Read the model definition and answer for the solid it produces. Units are mm, in the model's axes. Face numbers are marked on the shaded views. A direction names the side the tool comes from. Give positions to 0.01 mm unless a question says otherwise; leave off trailing zeros. Write each loop counter-clockwise with the first axis right and the second up, starting at its lowest first coordinate (ties: lowest second). Pieces come first, ordered by that corner, then holes. Notation, with made-up numbers: (3, -34) -> (45, -34) arc R16 ccw to (45, -7) -> close; hole circle Ø5 at (31, 82.5). An arc over 180 degrees is marked (long way). Use a Markdown table: item, result.
Autodesk Fusion 360 part; units mm, degrees
sketch "Sketch1" plane through (0, 0, 0) normal (0, 0, 1) x (1, 0, 0)
  line L0 (0, 0) -> (55, 0)
  line L1 (55, 0) -> (55, 50)
  line L2 (55, 50) -> (0, 50)
  line L3 (0, 50) -> (0, 0)
  dimension "d1" = 55
  dimension "d2" = 50
extrude "Extrude1" add sketch "Sketch1" along normal blind 5
sketch "Sketch2" plane through (0, 0, 5) normal (0, 0, 1) x (-1, 0, 0)
  line L0 (0, -50) -> (0, 0)
  line L1 (0, 0) -> (-55, 0)
  line L2 (-55, 0) -> (-55, -50)
  line L3 (-55, -50) -> (0, -50)
  circle A0 centre (-10, -40) radius 3
  circle A1 centre (-10, -10) radius 3
  circle A2 centre (-40, -10) radius 3
  circle A3 centre (-40, -40) radius 3
  dimension "d5" = 6
  dimension "d6" = 6
  dimension "d7" = 6
  dimension "d8" = 6
extrude "Extrude2" cut sketch "Sketch2" against normal blind 5 contours A0 | A1 | A2 | A3
sketch "Sketch3" plane through (0, 0, 5) normal (0, 0, 1) x (-1, 0, 0)
  circle A0 centre (-40, -40) radius 3
  circle A1 centre (-40, -10) radius 3
  circle A2 centre (-10, -40) radius 3
  circle A3 centre (-10, -10) radius 3
  line L0 (0, -50) -> (0, 0)
  line L1 (0, 0) -> (-55, 0)
  line L2 (-55, 0) -> (-55, -50)
  line L3 (-55, -50) -> (0, -50)
  circle A4 centre (-10, -10) radius 5
  circle A5 centre (-10, -40) radius 5
  circle A6 centre (-40, -40) radius 5
  circle A7 centre (-40, -10) radius 5
  dimension "d11" = 10
  dimension "d12" = 10
  dimension "d13" = 10
  dimension "d14" = 10
extrude "Extrude3" cut sketch "Sketch3" against normal blind 2 contours A4 | A5 | A6 | A7
sketch "Sketch4" plane through (0, 0, 5) normal (0, 0, 1) x (-1, 0, 0)
  circle A0 centre (-40, -40) radius 5
  circle A1 centre (-40, -10) radius 5
  circle A2 centre (-10, -40) radius 5
  circle A3 centre (-10, -10) radius 5
  line L0 (0, -50) -> (0, 0)
  line L1 (0, 0) -> (-55, 0)
  line L2 (-55, 0) -> (-55, -50)
  line L3 (-55, -50) -> (0, -50)
  line L4 (-50, 0) -> (-55, 0)
  line L5 (-55, 0) -> (-55, -50)
  line L6 (-55, -50) -> (-50, -50)
  line L7 (-50, -50) -> (-50, 0)
  dimension "d17" = 5
  dimension "d18" = 50
extrude "Extrude4" add sketch "Sketch4" along normal blind 50 contours L1 L2 L3 L4 L5 L6 L7
sketch "Sketch5" plane through (50, 0, 0) normal (-1, 0, 0) x (0, -1, 0)
  line L0 (-50, 5) -> (0, 5)
  line L1 (0, 5) -> (0, 55)
  line L2 (0, 55) -> (-50, 55)
  line L3 (-50, 55) -> (-50, 5)
  circle A0 centre (-40, 45) radius 3
  circle A1 centre (-10, 45) radius 3
  circle A2 centre (-10, 15) radius 3
  circle A3 centre (-40, 15) radius 3
  dimension "d21" = 6
  dimension "d22" = 6
  dimension "d23" = 6
  dimension "d24" = 6
extrude "Extrude5" cut sketch "Sketch5" against normal blind 5 contours A0 | A1 | A2 | A3
sketch "Sketch6" plane through (50, 0, 0) normal (-1, 0, 0) x (0, -1, 0)
  circle A0 centre (-10, 45) radius 3
  circle A1 centre (-10, 15) radius 3
  circle A2 centre (-40, 45) radius 3
  circle A3 centre (-40, 15) radius 3
  line L0 (-50, 5) -> (0, 5)
  line L1 (0, 5) -> (0, 55)
  line L2 (0, 55) -> (-50, 55)
  line L3 (-50, 55) -> (-50, 5)
  circle A4 centre (-40, 45) radius 5
  circle A5 centre (-10, 45) radius 5
  circle A6 centre (-40, 15) radius 5
  circle A7 centre (-10, 15) radius 5
  dimension "d27" = 10
  dimension "d28" = 10
  dimension "d29" = 10
  dimension "d30" = 10
extrude "Extrude6" cut sketch "Sketch6" against normal blind 2 contours A4 | A5 | A6 | A7
sketch "Sketch7" plane through (0, 0, 0) normal (0, -1, 0) x (1, 0, 0)
  line L0 (0, 0) -> (55, 0)
  line L1 (55, 0) -> (55, 55)
  line L2 (55, 55) -> (50, 55)
  line L3 (50, 55) -> (50, 5)
  line L4 (50, 5) -> (0, 5)
  line L5 (0, 5) -> (0, 0)
  line L6 (55, 0) -> (0, 0)
  line L7 (0, 0) -> (0, 55)
  line L8 (0, 55) -> (55, 55)
  line L9 (55, 55) -> (55, 0)
extrude "Extrude7" add sketch "Sketch7" against normal blind 5 contours L3 L4 L7 L8
sketch "Sketch8" plane through (0, 50, 0) normal (0, 1, 0) x (-1, 0, 0)
  line L0 (-55, 0) -> (0, 0)
  line L1 (0, 0) -> (0, 5)
  line L2 (0, 5) -> (-50, 5)
  line L3 (-50, 5) -> (-50, 55)
  line L4 (-50, 55) -> (-55, 55)
  line L5 (-55, 55) -> (-55, 0)
  line L6 (0, 55) -> (-55, 55)
  line L7 (-55, 55) -> (-55, 0)
  line L8 (-55, 0) -> (0, 0)
  line L9 (0, 0) -> (0, 55)
extrude "Extrude8" add sketch "Sketch8" against normal blind 5 contours L2 L3 L6 L9
sketch "Sketch9" plane through (0, 50, 0) normal (0, 1, 0) x (-1, 0, 0)
  line L0 (-55, 0) -> (0, 0)
  line L1 (0, 0) -> (0, 55)
  line L2 (0, 55) -> (-55, 55)
  line L3 (-55, 55) -> (-55, 0)
  circle A0 centre (0, 55) radius 50
extrude "Extrude9" cut sketch "Sketch9" against normal blind 50 contours L1 L2 A0 | L1 L2 A0
fillet "Fillet1" radius 5 4 edges at (0, 0, 2.5) (52.5, 0, 55) (52.5, 50, 55) (0, 50, 2.5)
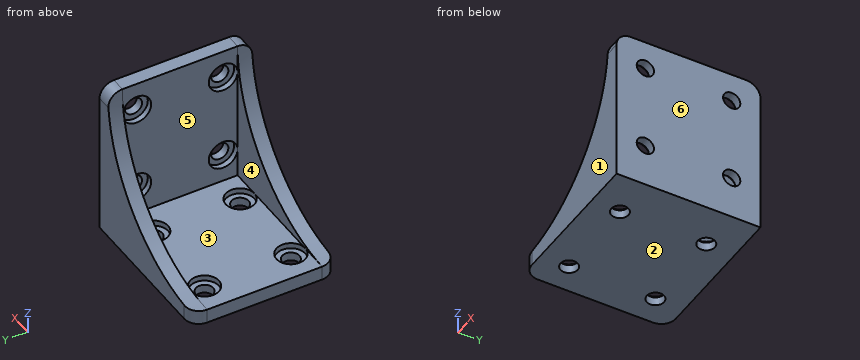
Item 1: For a pull along Y with two mould halves and no side action, classify the marked faces 1, 2, 3 and 4 as +Y half, -Y half, draft (parallel to the pull), parting line (faces both ways), or undercut.
Return value:
| item | result |
|---|---|
| face 1 | -Y half |
| face 2 | draft |
| face 3 | undercut |
| face 4 | undercut |
Item 2: Straight lines are drawn through the part: line 1 along Y through (x, z) = (10, 4.35); line 2 along Z through (x, y) = (51, 10); line 3 along Y through (x, z) = (40, 0.75). For each, find the intervals that lie inside material, in ascending order. Write a range as [from, to].
Return value:
| item | result |
|---|---|
| line 1 | [0, 5], [15, 35], [45, 50] |
| line 2 | [0, 10], [20, 40], [50, 55] |
| line 3 | [0, 7], [13, 37], [43, 50] |
Item 3: A cutting plane is placed at B-B (x = 41.5). Give the vertices of the cut face in (y, z).
Return value:
| item | result |
|---|---|
| outline | (0, 0) -> (7.4, 0) -> (7.4, 3) -> (5.23, 3) -> (5.23, 5) -> (5, 5) -> (5, 27.11) -> (0, 27.11) -> close; (12.6, 0) -> (37.4, 0) -> (37.4, 3) -> (35.23, 3) -> (35.23, 5) -> (14.77, 5) -> (14.77, 3) -> (12.6, 3) -> close; (42.6, 0) -> (50, 0) -> (50, 27.11) -> (45, 27.11) -> (45, 5) -> (44.77, 5) -> (44.77, 3) -> (42.6, 3) -> close |
Item 4: A cutting plane is placed at D-D (y = 10). Count the separate pieces of the cut face and the enclosed holes in it, then the cut area to 3 significant figures.
Return value:
| item | result |
|---|---|
| separate pieces | 5 |
| enclosed holes | 0 |
| area | 373 mm^2 |
Item 5: A cutting plane is placed at A-A (z = 14). Give the vertices of the cut face in (x, y), then the cut area to 3 significant figures.
Return value:
| item | result |
|---|---|
| outline | (28.62, 0) -> (55, 0) -> (55, 7.17) -> (52, 7.17) -> (52, 5.1) -> (50, 5.1) -> (50, 5) -> (28.62, 5) -> close; (28.62, 45) -> (50, 45) -> (50, 44.9) -> (52, 44.9) -> (52, 42.83) -> (55, 42.83) -> (55, 50) -> (28.62, 50) -> close; (50, 14.9) -> (52, 14.9) -> (52, 12.83) -> (55, 12.83) -> (55, 37.17) -> (52, 37.17) -> (52, 35.1) -> (50, 35.1) -> close |
| area | 391 mm^2 |
Item 6: Each of these flat-tipped pins is pushed along its axis until it touches: P1, Ø5, axis at x = 39.5, y = 12.5, coming from the +Z side; P2, Ø1.5, axis at x = 13.5, y = 9, coming from the +Z side; P3, Ø3.5, axis at x = 40, y = 40, coming from the +Z side; P4, Ø10, axis at y = 31.5, z = 13.5, coming from the -X side. Where does it stop, or does it pass through?
Return value:
| item | result |
|---|---|
| P1 | z = 5 |
| P2 | z = 3 |
| P3 | through |
| P4 | x = 50 |
Item 7: A tool of negligible diameter and unlimited length cuts with its end or side. For the marked faces 5 and 6, from which of +Z, -Z, +X, -X, +Y, -Y can it reach the whole face along a straight path? Write none if from no direction.
Return value:
| item | result |
|---|---|
| face 5 | +Z, -X |
| face 6 | +Z, -Z, +X, +Y, -Y |
Item 8: A cutting plane is placed at C-C (y = 21.5). Give the vertices of the cut face in (x, z), then the cut area to 3 significant figures.
Return value:
| item | result |
|---|---|
| outline | (0, 0) -> (55, 0) -> (55, 55) -> (50, 55) -> (50, 5) -> (0, 5) -> close |
| area | 525 mm^2 |
